The model under review builds one solid part; all positions refer to its coordinate system, in mm. Face numbers are marked on the shaded views. Round coordinates to 2 decimals unless told otherwise and drop trailing zeros. Order: outer loops, then holes, each group sorted by start corner. A loop starts at its lowest first (then second) coordinate and runs counter-clockwise, first axis right, second up. Notation, with made-up numbers: M -38.75,69.25 L 13.25,69.25 A27 cw 13.25,106.25 Z; hole C 36.5,-17 d9. An arc over 180 degrees is marked long. Use a Markdown table: item, result. Add a question column.
1. Consider section C-C on x = -15.25. State the section outline as (y, z) points, then the cut area to 3 significant figures.
2. The part is to be moulded in two halves that separate along Y. For the marked faces 1, 2 and 3, say which applies: +Y half, -Y half, draft (parallel to the pull), parting line (faces both ways), or undercut.
3. To check wall thickness, follow probe 1 along Z at (x, y) = (-12.5, 0); probe 2 along Z at (x, y) = (-15.5, 23); probe 3 along Z at (x, y) = (-1.3, 0). State the ranges of each line that lie inside material, in increasing order.
4. Consider section B-B on y = -48. State the section outline as (x, z) points, then the cut area to 3 significant figures.
5. Insertion check: P1, Ø10, axis at x = -13, z = -15.5, coming from the +Y side; P2, Ø8, axis at x = -5.5, z = 2, coming from the -Y side; P3, Ø4, axis at x = -4, z = -24, coming from the -Y side; P4, Ø8, axis at y = -48, z = 0, coming from the +X side. Each pin has a flat end and moves straight along its axis. Give the tip position at first contact, or say it passes through.
6. Consider section A-A on z = 0. State the section outline as (x, y) points.
from build123d import *

# Parameters (mm, degrees)
F2_SIZE          = 1
F3_R             = 2.5
F4_DEPTH         = 20.001
F4_COPIES_COUNT  = 3
F4_COPIES_ANGLE  = 120
F4_COPIES1_COUNT = 3
F4_COPIES1_ANGLE = 120
F5_R             = 2.5
F6_DEPTH         = 20.001


# Not quite as in the source:
# - a pattern or mirror of a feature is missing from the dataset's text; its kind, count and spacing are read off the source's solid


with BuildPart() as f1:
    # F0 (on Front) → F1 (revolve)
    with BuildSketch(Plane.XZ):
        Polygon((-4, 38.6), (0, 38.6), (0, 55), (-20, 55), (-20, 40), (-10.5399421904, 40), (-4, 39.6), align=None)
    revolve(axis=Axis((12.3917190358, 0, 0), (1, 0, 0)))

    # F2
    f2_edges = [f1.edges().sort_by_distance(p)[0] for p in [
        (-20, 0, -40),
    ]]
    chamfer(f2_edges, length=F2_SIZE)

    # F3 (on face) → F4 (cut, through all)
    with BuildSketch(Plane(origin=(-20, 0, 0), x_dir=(0, -1, 0), z_dir=(-1, 0, 0))):
        with Locations((48, 0)):
            Circle(F3_R)
    f4 = extrude(amount=-F4_DEPTH, mode=Mode.SUBTRACT)

    # F4_copies: F4 ×3 about axis
    f4_copies_axis = Axis((0, 0, 0), (1, 0, 0))
    for i in range(1, F4_COPIES_COUNT):
        add(f4.rotate(f4_copies_axis, i * F4_COPIES_ANGLE / (F4_COPIES_COUNT - 1)), mode=Mode.SUBTRACT)

    # F4_copies1: F4 ×3 about axis
    f4_copies1_axis = Axis((0, 0, 0), (-1, 0, 0))
    for i in range(1, F4_COPIES1_COUNT):
        add(f4.rotate(f4_copies1_axis, i * F4_COPIES1_ANGLE / (F4_COPIES1_COUNT - 1)), mode=Mode.SUBTRACT)

    # F5 (on face) → F6 (cut, through all)
    with BuildSketch(Plane(origin=(-20, 0, 0), x_dir=(0, -1, 0), z_dir=(-1, 0, 0))):
        with Locations((-48, 0)):
            Circle(F5_R)
    extrude(amount=-F6_DEPTH, mode=Mode.SUBTRACT)


solid = f1.part
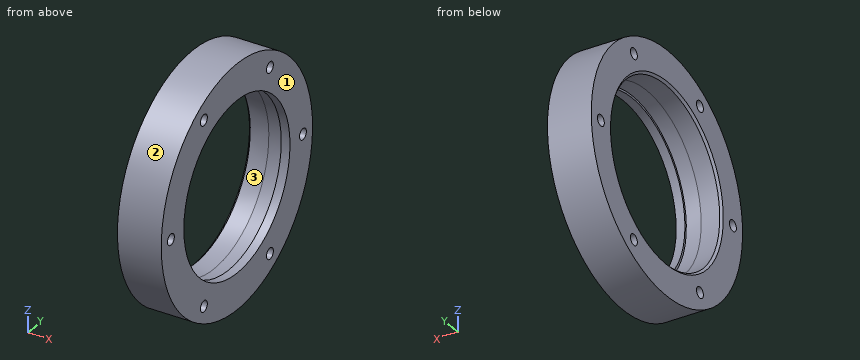
Answer block:
| question | item | result |
|---|---|---|
| 1 | outline | C 0,0 d110; hole C -48,0 d5; hole C 0,0 d80; hole C -24,-41.57 d5; hole C -24,41.57 d5; hole C 24,-41.57 d5; hole C 24,41.57 d5; hole C 48,0 d5 |
| 1 | area | 4,360 mm^2 |
| 2 | face 1 | draft |
| 2 | face 2 | parting line |
| 2 | face 3 | undercut |
| 3 | probe 1 | -55 to -40, 40 to 55 |
| 3 | probe 2 | -49.96 to -43.86, -39.28 to -32.73, 32.73 to 39.28, 43.86 to 49.96 |
| 3 | probe 3 | -55 to -38.6, 38.6 to 55 |
| 4 | outline | M -20,-26.85 L 0,-26.85 L 0,-2.5 L -20,-2.5 Z; M -20,2.5 L 0,2.5 L 0,26.85 L -20,26.85 Z |
| 4 | area | 974 mm^2 |
| 5 | P1 | y = 53.99 |
| 5 | P2 | y = -55 |
| 5 | P3 | y = -50.41 |
| 5 | P4 | x = 0 |
| 6 | outline | M -20,-55 L 0,-55 L 0,-50.5 L -20,-50.5 Z; M -20,-45.5 L 0,-45.5 L 0,-38.6 L -4,-38.6 L -4,-39.6 L -10.54,-40 L -19,-40 L -20,-41 Z; M -20,41 L -19,40 L -10.54,40 L -4,39.6 L -4,38.6 L 0,38.6 L 0,45.5 L -20,45.5 Z; M -20,50.5 L 0,50.5 L 0,55 L -20,55 Z |
